Check sheet for the modelled part. Datum: model origin and axes. Units: mm. A direction names the side the tool comes from. Round coordinates to 2 decimals unless told otherwise and drop trailing zeros. Order: outer loops, then holes, each group sorted by start corner. A loop starts at its lowest first (then second) coordinate and runs counter-clockwise, first axis right, second up.
Q1. Cross-section at C-C on y = 65.5. Record the cut outline in (x, z).
Q2. Mould release check, pull along X, two halves, no side actions. Record for faces 1 (the flat face through (-300, 35, 20)), 2 (the flat face through (-30, 50, 20)), 3 (the flat face through (-277, 70, 15)), 4 (the cylindrical face through (-116.034, 24.65, 20.521)): +X half, -X half, draft (parallel to the pull), parting line (faces both ways), or undercut.
Q3. Scan lines: probe 1 along X at (y, z) = (38, 20); probe 2 along Z at (x, y) = (-270, 321.5); probe 3 along X at (y, z) = (182, 9). Record each from-to range of solid material in increasing order.
Q4. Cross-section at B-B on z = 20. Record the cut outline in (x, y), then the cut area to 3 significant figures.
Q5. Cross-section at A-A on x = -270. Record the cut outline in (y, z).
Q6. Depth check by flat-ended pin: P1, Ø1.5, axis at y = 155.5, z = 11.5, coming from the -X side; P2, Ø4, axis at x = -118.5, z = 19.5, coming from the -Y side; P3, Ø5, axis at x = -271.5, z = 22, coming from the +Y side. Enter the tip coordinate at first touch or a pass-through.
Q7. Cross-section at D-D on x = -120. Record the cut outline in (y, z), then the cut area to 3 significant figures.
Q8. Set-up check for faces 5 (the flat face through (0, 177, 20)), 6 (the cylindrical face through (-264.1, 330.3, 25.4)), 7 (the flat face through (-240, 188, 20)), 8 (the flat face through (-120, 50, 20)), 9 (the flat face through (-115, 177, 40)): record each of +Z, -Z, +X, -X, +Y, -Y from which the full face is reachable in a straight line by a thin tool's end or side.
from build123d import *

# Parameters (mm, degrees)
EXTRUDE_1_DEPTH     = 40
SKETCH_2_R          = 8
CUT_EXTRUDE_1_DEPTH = 300
SKETCH_3_R          = 4
CUT_EXTRUDE_2_DEPTH = 50


with BuildPart() as part:
    # Эскиз1 → Бобышка-Вытянуть1 (new body)
    with BuildSketch(Plane.XY):
        Polygon((-300, 310), (-300, 350), (0, 350), (0, 0), (-300, 0), (-300, 70), (-240, 70), (-240, 310), align=None)
    extrude(amount=EXTRUDE_1_DEPTH)

    # Эскиз2 → Вырез-Вытянуть1 (cut)
    with BuildSketch(Plane(origin=(0, 350, 0), x_dir=(1, 0, 0), z_dir=(0, 1, 0))):
        with Locations(Location((-270, -20, 0), (0, 0, 180))):
            Circle(SKETCH_2_R)
    extrude(amount=-CUT_EXTRUDE_1_DEPTH, mode=Mode.SUBTRACT)

    # Эскиз3 → Вырез-Вытянуть2 (cut)
    with BuildSketch(Plane.XZ):
        with Locations(Location((-30, 20, 0), (0, 0, 270))):
            Circle(SKETCH_3_R)
        with Locations(Location((-120, 20, 0), (0, 0, 270))):
            Circle(SKETCH_3_R)
        with Locations(Location((-210, 20, 0), (0, 0, 270))):
            Circle(SKETCH_3_R)
    extrude(amount=-CUT_EXTRUDE_2_DEPTH, mode=Mode.SUBTRACT)


solid = part.part
Results found:
1. outline: (-300, 0) - (0, 0) - (0, 40) - (-300, 40) - close; hole circle Ø16 at (-270, 20)
2. face 1: -X half
2. face 2: undercut
2. face 3: draft
2. face 4: undercut
3. probe 1: x = -300 to -214, -206 to -124, -116 to -34, -26 to 0
3. probe 2: z = 0 to 12, 28 to 40
3. probe 3: x = -240 to 0
4. outline: (-300, 0) - (-214, 0) - (-214, 50) - (-206, 50) - (-206, 0) - (-124, 0) - (-124, 50) - (-116, 50) - (-116, 0) - (-34, 0) - (-34, 50) - (-26, 50) - (-26, 0) - (0, 0) - (0, 350) - (-262, 350) - (-262, 310) - (-240, 310) - (-240, 70) - (-262, 70) - (-262, 50) - (-278, 50) - (-278, 70) - (-300, 70) - close; (-300, 310) - (-278, 310) - (-278, 350) - (-300, 350) - close
4. area: 88,400 mm2
5. outline: (0, 0) - (70, 0) - (70, 12) - (50, 12) - (50, 28) - (70, 28) - (70, 40) - (0, 40) - close; (310, 0) - (350, 0) - (350, 12) - (310, 12) - close; (310, 28) - (350, 28) - (350, 40) - (310, 40) - close
6. P1: stops at x = -240
6. P2: stops at y = 50
6. P3: stops at y = 50
7. outline: (0, 0) - (350, 0) - (350, 40) - (0, 40) - (0, 24) - (50, 24) - (50, 16) - (0, 16) - close
7. area: 13,600 mm2
8. face 5: +Z, -Z, +X, +Y, -Y
8. face 6: +Y
8. face 7: +Z, -Z, -X
8. face 8: -Y
8. face 9: +Z, +X, -X, +Y, -Y
